Read the model definition and answer for the solid it produces. Units are mm, in the model's axes. A direction names the side the tool comes from. Coordinates: 2 decimals unless noted, no trailing zeros. Order: outer loops, then holes, each group sorted by start corner. A loop starts at its lowest first (then second) coordinate and runs counter-clockwise, first axis right, second up.
```python
from build123d import *

# Parameters (mm, degrees)
F0_W      = 88
F0_H      = 37
F1_DEPTH  = 1.75
F2_W      = 82.3
F2_H      = 29.5
F3_DEPTH  = 1.5
F4_R      = 4
F5_DEPTH  = 10
F6_R      = 4
F7_R      = 1.35
F8_DEPTH  = 88.001
F9_R      = 3
F10_DEPTH = 25


with BuildPart() as f1:
    # F0 (on Top) → F1 (new body)
    with BuildSketch(Plane.XY):
        with Locations((-44, 18.5)):
            Rectangle(F0_W, F0_H)
    extrude(amount=F1_DEPTH)

    # F2 (on face) → F3 (join)
    with BuildSketch(Plane.XY.offset(1.75)):
        with Locations((-43.1, 18.5)):
            Rectangle(F2_W, F2_H)
    extrude(amount=F3_DEPTH)

    # F4 (on face) → F5 (join)
    with BuildSketch(Plane(origin=(0, 0, 0), x_dir=(1, 0, 0), z_dir=(0, 0, -1))):
        with Locations((-53.5, -17.5)):
            Circle(F4_R)
        with Locations((-34.5, -17.5)):
            Circle(F4_R)
    extrude(amount=F5_DEPTH)

    # F6
    f6_edges = [f1.edges().sort_by_distance(p)[0] for p in [
        (-57.5, 17.5, -10),
        (-38.5, 17.5, -10),
    ]]
    fillet(f6_edges, radius=F6_R)

    # F7 (on face) → F8 (cut, through all)
    with BuildSketch(Plane.YZ):
        with Locations((17.5, -3.85)):
            Circle(F7_R)
    extrude(amount=-F8_DEPTH, mode=Mode.SUBTRACT)

    # F9
    f9_edges = [f1.edges().sort_by_distance(p)[0] for p in [
        (-88, 0, 0.875),
        (-88, 37, 0.875),
        (0, 37, 0.875),
        (0, 0, 0.875),
    ]]
    fillet(f9_edges, radius=F9_R)

    # F2 (on face) → F10 (intersect)
    with BuildSketch(Plane.XY.offset(1.75)):
        with Locations((-43.1, 18.5)):
            Rectangle(F2_W, F2_H)
    extrude(amount=-F10_DEPTH, mode=Mode.INTERSECT)


solid = f1.part
```
1) A cutting plane is placed at D-D, the plane y = 29.5. Determine the outline of the cut face in (x, z), and give its area (3 significant figures).
A:
outline: (-84.25, 0) - (-1.95, 0) - (-1.95, 1.75) - (-84.25, 1.75) - close
area: 144 mm2
2) Straight lines are drawn through the part: line 1 (Z direction, x = -53.75, y = 17.5); line 2 (Z direction, x = -38.5, y = 19.5); line 3 (Z direction, x = -33, y = 17.5). For each, find the intervals that lie inside material, in ascending order.
A:
line 1: z = -9.99 to -5.2, -2.5 to 1.75
line 2: z = 0 to 1.75
line 3: z = -9.71 to -5.2, -2.5 to 1.75
3) Which of the six approach directions +Z, -Z, +X, -X, +Y, -Y give full straight-line access (tool end or side, diameter ignored) to faces 4 (the flat face through (-44, 33.25, 1)), 5 (the cylindrical face through (-30.805, 19.032, -2.958))?
A:
face 4: +Z, -Z, +X, -X, +Y
face 5: -Z
4) A cutting plane is placed at A-A, the plane y = 17.5. Determine the outline of the cut face in (x, z).
A:
outline: (-84.25, 0) - (-57.5, 0) - (-57.5, -2.5) - (-49.5, -2.5) - (-49.5, 0) - (-38.5, 0) - (-38.5, -2.5) - (-30.5, -2.5) - (-30.5, 0) - (-1.95, 0) - (-1.95, 1.75) - (-84.25, 1.75) - close; (-57.5, -6) arc R4 ccw to (-49.5, -6) - (-49.5, -5.2) - (-57.5, -5.2) - close; (-38.5, -6) arc R4 ccw to (-30.5, -6) - (-30.5, -5.2) - (-38.5, -5.2) - close
5) Flat-ended cylindrical pins translate along their axes: pin 1 Ø8 at (x, y) = (-56.5, 22.5) entering from -Z; pin 2 Ø3.5 at (y, z) = (17.5, -3.85) entering from -X; pin 3 Ø5 at (x, y) = (-17, 22) entering from -Z. Find the tip coordinate at first contact, or state that the pin passes through.
A:
pin 1: stops at z = -9.56
pin 2: stops at x = -57.5
pin 3: stops at z = 0
6) A cutting plane is placed at C-C, the plane z = -3.85. Determine the outline of the cut face in (x, y).
A:
outline: (-57.27, 16.15) arc R4 ccw to (-49.73, 16.15) - close; (-57.27, 18.85) - (-49.73, 18.85) arc R4 ccw to start; (-38.27, 16.15) arc R4 ccw to (-30.73, 16.15) - close; (-38.27, 18.85) - (-30.73, 18.85) arc R4 ccw to start
7) Determine the mould class of faces 1 (the cylindrical face through (-34.445, 17.324, -2.511)), 2 (the flat face through (-44, 19, 1.75)), 3 (the flat face through (-44, 3.75, 1)) for opening direction Z: pulls with the +Z half, pulls with the -Z half, needs draft (parallel to the pull), parting line crosses it, or undercut.
A:
face 1: undercut
face 2: pulls with the +Z half
face 3: needs draft
8) A cutting plane is placed at B-B, the plane x = -53.5. Determine the outline of the cut face in (y, z).
A:
outline: (3.75, 0) - (13.5, 0) - (13.5, -6) arc R4 ccw to (21.5, -6) - (21.5, 0) - (33.25, 0) - (33.25, 1.75) - (3.75, 1.75) - close; hole circle Ø2.7 at (17.5, -3.85)
